Drawing for the job (mm, zero at the part's lowest x, y, z). Give positions to 0.01 mm unless a question says otherwise; leave off trailing zeros. Write each loop counter-clockwise with the first axis right and the second up, starting at its lowest first coordinate (ties: lowest second). Pieces come first, ordered by that corner, then holes. Notation, with made-up numbers: M 37.5,79 L 73.5,79 A18 cw 73.5,93 Z; hole C 75.5,-32 d10. An arc over 180 degrees is marked long. Answer as a JSON object with one key per item and string values. Group by question number.
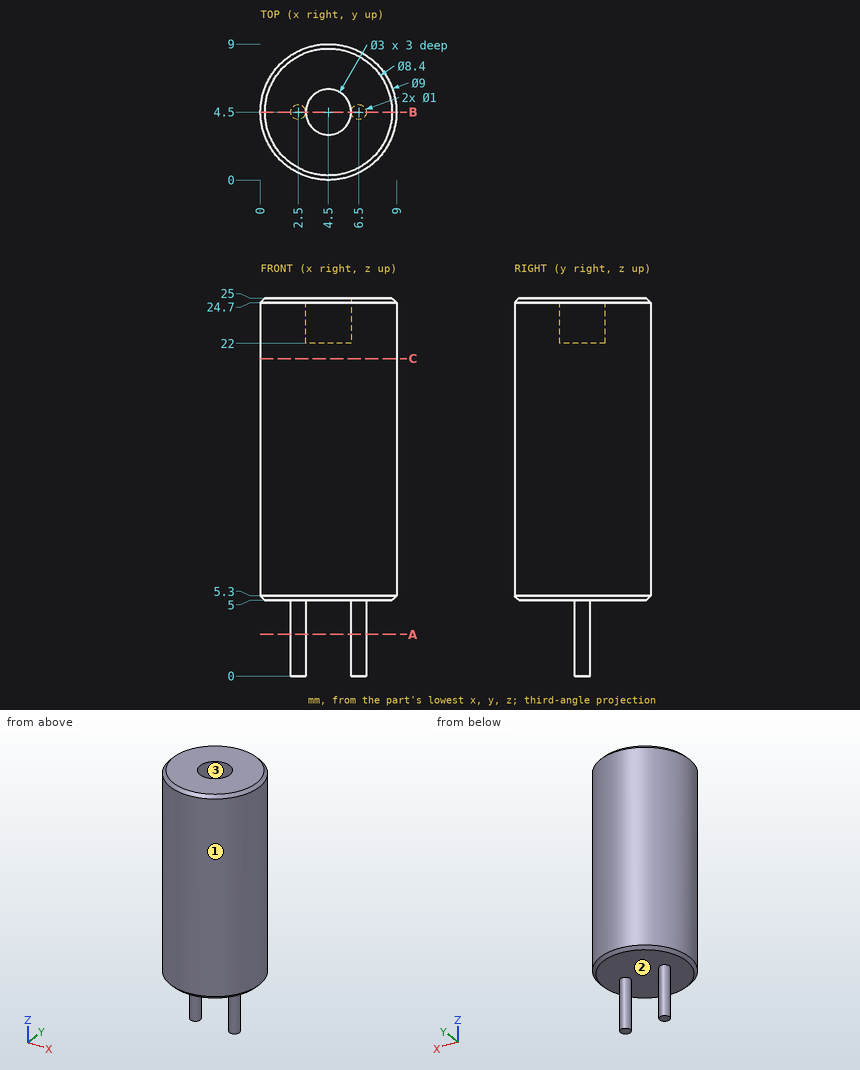
Q1. Slice it at B-B, the plane y = 4.5. Write the cut outline in (x, z).
Q2. Slice it at A-A, the plane z = 2.75. Write the cut outline in (x, y), then the cut area to 3 significant figures.
Q3. Slice it at C-C, the plane z = 21. Write the cut outline in (x, y), then the cut area to 3 significant figures.
Q4. Two-plate mould, pull along Y, no slides. Class the marked faces 1, 2 and 3: +Y half, -Y half, draft (parallel to the pull), parting line (faces both ways), or undercut.
Q5. Wall check: L1, parallel to Y at x = 4.5, z = 23.05; L2, parallel to Z at x = 7.5, y = 6.5; L3, parallel to Y at x = 5, z = 22.5. Give the ranges that are in metal, low to high.
Q6. Drop flat-ended pins along their axis: P1, Ø3, axis at y = 6, z = 19, coming from the -X side; P2, Ø1.5, axis at x = 8, z = 4.5, coming from the +Y side; P3, Ø1.5, axis at x = 5, y = 5, coming from the +Z side; P4, Ø2, axis at y = 6.5, z = 9, coming from the +X side. Give the stop position or say it passes through.
Solved:
{
 "1": {"outline": "M 0,5.3 L 0.3,5 L 2,5 L 2,0 L 3,0 L 3,5 L 6,5 L 6,0 L 7,0 L 7,5 L 8.7,5 L 9,5.3 L 9,24.7 L 8.7,25 L 6,25 L 6,22 L 3,22 L 3,25 L 0.3,25 L 0,24.7 Z"},
 "2": {"outline": "C 2.5,4.5 d1; C 6.5,4.5 d1", "area": "1.57 mm²"},
 "3": {"outline": "C 4.5,4.5 d9", "area": "63.6 mm²"},
 "4": {"face 1": "parting line", "face 2": "draft", "face 3": "undercut"},
 "5": {"L1": "y = 0 to 3, 6 to 9", "L2": "z = 5 to 25", "L3": "y = 0.03 to 3.09, 5.91 to 8.97"},
 "6": {"P1": "stops at x = 0", "P2": "stops at y = 7.53", "P3": "stops at z = 22", "P4": "stops at x = 8.89"}
}
